Autodesk Inventor part; units mm, degrees
ref_plane "YZ Plane" through (0, 0, 0) normal (1, 0, 0) x (0, 1, 0)
ref_plane "XZ Plane" through (0, 0, 0) normal (0, 1, 0) x (-1, 0, 0)
ref_plane "XY Plane" through (0, 0, 0) normal (0, 0, 1) x (1, 0, 0)
sketch "Esquisse1" plane through (0, 0, 0) normal (0, 1, 0) x (-1, 0, 0)
  circle A0 centre (0, 0) radius 45
  dimension "d0" = 90
extrude "Extrusion1" add sketch "Esquisse1" along normal blind 27.3
fillet "Congé1" radius 1 1 edges at (45, 27.3, 0)
sketch "Esquisse2" plane through (0, 27.3, 0) normal (0, 1, 0) x (1, 0, 0)
  circle A0 centre (0, 0) radius 44
  circle A1 centre (0, 0) radius 20
  dimension "d4" = 40
extrude "Extrusion2" add sketch "Esquisse2" along normal blind 2.3 contours A1
fillet "Congé2" radius 0.5 1 edges at (-20, 29.6, 0)
sketch "Esquisse3" plane through (0, 0, 0) normal (0, -1, 0) x (1, 0, 0)
  circle A0 centre (0, 0) radius 45
  circle A1 centre (0, 0) radius 12.5
  dimension "d8" = 25
extrude "Extrusion3" add sketch "Esquisse3" along normal blind 3.2 contours A1
sketch "Esquisse5" plane through (0, -3.2, 0) normal (0, -1, 0) x (1, 0, 0)
  circle A0 centre (0, 0) radius 12.5
  circle A1 centre (0, 0) radius 5
  dimension "d11" = 10
extrude "Extrusion4" add sketch "Esquisse5" along normal blind 22 contours A1
sketch "Esquisse6" plane through (0, 0, 0) normal (0, -1, 0) x (1, 0, 0)
  circle A0 centre (0, 0) radius 12.5
  circle A1 centre (0, 24) radius 2.5
  dimension "d14" = 5
  dimension "d15" = 24
extrude "Extrusion5" cut sketch "Esquisse6" against normal blind 6 contours A1
pattern_circular "Réseau circulaire1" count 3 over 360 about axis through (0, 0, 0) along (0, -1, 0) of "Extrusion5"
properties part number "Moteur MAxon" material "Acier inoxydable"
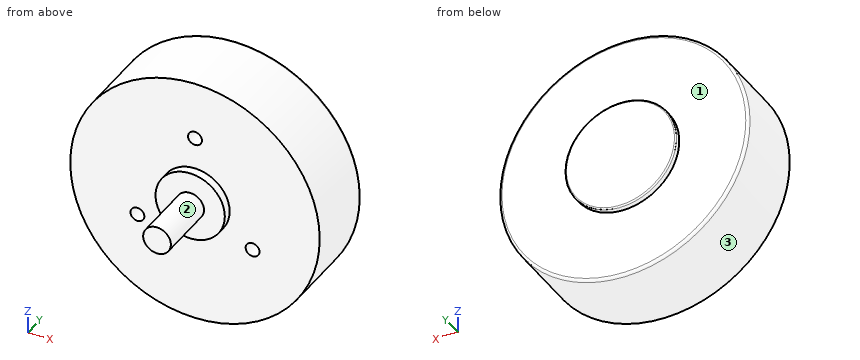
Work out the finished part from the listing and answer in its coordinate system (mm). Face numbers are marked on the shaded views. A direction names the side the tool comes from. Round coordinates to 2 decimals unless told otherwise and drop trailing zeros. Write each loop counter-clockwise with the first axis right and the second up, starting at its lowest first coordinate (ties: lowest second). Pieces come first, ordered by that corner, then holes. Notation, with made-up numbers: (28.5, 7) - (35.5, 7) arc R15 cw to (35.5, 19) - close; hole circle Ø3 at (-27, -22). An arc over 180 degrees is marked (long way). Return JSON: item names as keys, results as strings. Group by question number.
Q1. Find the intervals of material crossed by L1, parallel to Z at x = 0, y = 2; L2, parallel to Y at x = 14, z = -40.5; L3, parallel to Y at x = -10.5, z = -6, in increasing order.
Q2. Each of these flat-tipped pins is pushed along its axis until it touches: pin 1 Ø8 at (x, z) = (29.5, 6) entering from -Y; pin 2 Ø1.5 at (x, z) = (-20, -11.5) entering from -Y; pin 3 Ø6.5 at (x, z) = (-20.78, -12) entering from +Y. Where does it stop, or does it pass through?
Q3. The part is cut by section A-A on z = 0. Write down the section's boundary in (x, y), then the cut area to 3 significant figures.
Q4. The part is cut by section B-B on x = 0. Write down the section's boundary in (y, z), then the cut area to 3 significant figures.
Q5. For the marked faces 1, 2 and 3, determine the directions among +Z, -Z, +X, -X, +Y, -Y from which every point of the face is accessible in a straight line to the end or side of a thin tool.
Q6. The part is cut by section C-C on y = 19.5. Write down the section's boundary in (x, z), then the cut area to 3 significant figures.
Q7. The part is cut by section D-D on y = 2.5. Write down the section's boundary in (x, z).
Solved:
{
 "1": {"L1": "-45 to 21.5, 26.5 to 45", "L2": "0 to 27.3", "L3": "-3.2 to 29.6"},
 "2": {"pin 1": "y = 0", "pin 2": "y = 6", "pin 3": "y = 27.3"},
 "3": {"outline": "(-45, 0) - (-12.5, 0) - (-12.5, -3.2) - (-5, -3.2) - (-5, -25.2) - (5, -25.2) - (5, -3.2) - (12.5, -3.2) - (12.5, 0) - (45, 0) - (45, 26.3) arc R1 ccw to (44, 27.3) - (20, 27.3) - (20, 29.1) arc R0.5 ccw to (19.5, 29.6) - (-19.5, 29.6) arc R0.5 ccw to (-20, 29.1) - (-20, 27.3) - (-44, 27.3) arc R1 ccw to (-45, 26.3) - close", "area": "2,850 mm²"},
 "4": {"outline": "(-25.2, -5) - (-3.2, -5) - (-3.2, -12.5) - (0, -12.5) - (0, -45) - (26.3, -45) arc R1 ccw to (27.3, -44) - (27.3, -20) - (29.1, -20) arc R0.5 ccw to (29.6, -19.5) - (29.6, 19.5) arc R0.5 ccw to (29.1, 20) - (27.3, 20) - (27.3, 44) arc R1 ccw to (26.3, 45) - (0, 45) - (0, 26.5) - (6, 26.5) - (6, 21.5) - (0, 21.5) - (0, 12.5) - (-3.2, 12.5) - (-3.2, 5) - (-25.2, 5) - close", "area": "2,820 mm²"},
 "5": {"face 1": "+Y", "face 2": "-Y", "face 3": "+Y, -Y"},
 "6": {"outline": "circle Ø90 at (0, 0)", "area": "6,360 mm²"},
 "7": {"outline": "circle Ø90 at (0, 0); hole circle Ø5 at (-20.78, -12); hole circle Ø5 at (0, 24); hole circle Ø5 at (20.78, -12)"}
}
